The model under review builds one solid part; all positions refer to its coordinate system, in mm. Coordinates: 2 decimals unless noted, no trailing zeros. Loops run counter-clockwise (first coordinate to the right, second up) from the corner with the lowest first, then second, coordinate; pieces in that order, holes last. Notation, with made-up numbers: M 43.25,-38.75 L 66.25,-38.75 A35 ccw 66.25,-0.75 Z; hole C -36,64.25 d5. An arc over 180 degrees is marked long. Return JSON: item names as keys, results as strings.
```python
from build123d import *

# Parameters (mm, degrees)
SKETCH1_W            = 90
SKETCH1_H            = 65
BOSS_EXTRUDE1_DEPTH  = 4.7625
M3_CLEARANCE_HOLE1_D = 3.4
M3_CLEARANCE_HOLE2_D = 3.4


with BuildPart() as part:
    # Sketch1 → Boss-Extrude1 (new body)
    with BuildSketch(Plane(origin=(0, 0, 0), x_dir=(1, 0, 0), z_dir=(0, 1, 0))):
        with Locations((45, 32.5)):
            Rectangle(SKETCH1_W, SKETCH1_H)
    extrude(amount=BOSS_EXTRUDE1_DEPTH)

    # M3 Clearance Hole1 (through all)
    with Locations(Plane(origin=(0, 4.7625, 0), x_dir=(1, 0, 0), z_dir=(0, 1, 0))):
        with Locations((36.709, 5.709), (36.709, 36.709), (5.709, 36.709), (5.709, 5.709)):
            Hole(M3_CLEARANCE_HOLE1_D / 2)

    # M3 Clearance Hole2 (through all)
    with Locations(Plane(origin=(0, 0, 0), x_dir=(-1, 0, 0), z_dir=(0, -1, 0))):
        with Locations((-17.5, 55), (-52.5, 55), (-80, 35), (-80, 10)):
            Hole(M3_CLEARANCE_HOLE2_D / 2)


solid = part.part
```
1. Add section D-D on x = 36. Give the boundary of the cut face in (y, z), plus the area to 3 significant figures.
Check values:
{"outline": "M 0,-65 L 4.76,-65 L 4.76,-38.25 L 0,-38.25 Z; M 0,-35.16 L 4.76,-35.16 L 4.76,-7.25 L 0,-7.25 Z; M 0,-4.16 L 4.76,-4.16 L 4.76,0 L 0,0 Z", "area": "280 mm²"}
2. The part is to be moulded in two halves that separate along X. For faces 1 (the face through (90, 2, -32)), 2 (the face through (0, 2, -32)), 3 (the face through (44, 2, 0)), 4 (the face through (6.08, 2.35, -4.05)), say which applies: released by +X, released by -X, zero draft, split by the parting line, or undercut.
Check values:
{"face 1": "released by +X", "face 2": "released by -X", "face 3": "zero draft", "face 4": "undercut"}
3. Add section A-A on x = 80. Give the boundary of the cut face in (y, z).
Check values:
{"outline": "M 0,-65 L 4.76,-65 L 4.76,-36.7 L 0,-36.7 Z; M 0,-33.3 L 4.76,-33.3 L 4.76,-11.7 L 0,-11.7 Z; M 0,-8.3 L 4.76,-8.3 L 4.76,0 L 0,0 Z"}
4. Add section B-B on z = -10. Give the boundary of the cut face in (x, y), plus the area to 3 significant figures.
Check values:
{"outline": "M 0,0 L 78.3,0 L 78.3,4.76 L 0,4.76 Z; M 81.7,0 L 90,0 L 90,4.76 L 81.7,4.76 Z", "area": "412 mm²"}
5. To check wall thickness, follow line 1 (Z direction, x = 80, y = 3.15); line 2 (X direction, y = 3.75, z = -55); line 3 (Z direction, x = 17.5, y = 3.45). State the ranges of each line that lie inside material, in increasing order.
Check values:
{"line 1": "-65 to -36.7, -33.3 to -11.7, -8.3 to 0", "line 2": "0 to 15.8, 19.2 to 50.8, 54.2 to 90", "line 3": "-65 to -56.7, -53.3 to 0"}
6. Add section C-C on x = 52.5. Give the boundary of the cut face in (y, z), plus the area to 3 significant figures.
Check values:
{"outline": "M 0,-65 L 4.76,-65 L 4.76,-56.7 L 0,-56.7 Z; M 0,-53.3 L 4.76,-53.3 L 4.76,0 L 0,0 Z", "area": "293 mm²"}
7. Insertion check: pin 1 Ø1 at (x, y) = (50.5, 2.5) entering from +Z. The pin has a flat end and moves straight along its axis. Give the tip position at first contact, or say it passes through.
Check values:
{"pin 1": "z = 0"}
